Geometry check sheet. Reference: the model listing, model coordinates, mm. Face numbers are marked on the shaded views. A direction names the side the tool comes from. Round coordinates to 2 decimals unless told otherwise and drop trailing zeros. Order: outer loops, then holes, each group sorted by start corner. A loop starts at its lowest first (then second) coordinate and runs counter-clockwise, first axis right, second up.
(1) Set-up check for the marked faces 1 and 2: record each of +Z, -Z, +X, -X, +Y, -Y from which the full face is reachable in a straight line by a thin tool's end or side.
(2) Cross-section at C-C on x = -1. Enter the section's corners in (y, z) (3 decimals).
(3) Thickness scan on L1, parallel to Y at x = -2, z = -22.5 (3 decimals); L2, parallel to X at y = 26, z = -34; L3, parallel to Y at x = 6.25, z = -3.5 (3 decimals). Record the ranges inside material, lowest first.
(4) Gauge pin test, flat ends, axial feed: P1, Ø3.5, axis at y = 2.5, z = -10, coming from the -X side; P2, Ø5, axis at x = 7.5, z = -17, coming from the +Y side (3 decimals); P3, Ø10, axis at y = 6, z = -12.5, coming from the +X side. Record the tip position at first contact, or that the pin passes through.
(5) Cross-section at A-A on z = -11. Enter the section's corners in (x, y) (3 decimals), and give its area (3 significant figures).
(6) Draft check along X on the marked faces 3, 4 and 5. Enter one of: pulls with the +X half, pulls with the -X half, needs draft (parallel to the pull), parting line crosses it, or undercut.
from build123d import *
from build123d.topology import SkipClean

# Parameters (mm, degrees)
SKETCH1_W               = 12.7
SKETCH1_H               = 25.4
BOSS_EXTRUDE1_DEPTH     = 3.175
SKETCH17_W              = 12.7
SKETCH17_H              = 3.175
BOSS_EXTRUDE5_DEPTH     = 31.75
F_3_8_CLEARANCE_HOLE1_D = 10.31748
BOSS_EXTRUDE6_DEPTH     = 3.175
CUT_EXTRUDE4_DEPTH      = 52.789749346
SKETCH31_W              = 2.00025
SKETCH31_H              = 25.4
BOSS_EXTRUDE9_DEPTH     = 18.034
CUT_EXTRUDE6_DEPTH      = 54.550805677
CUT_EXTRUDE6_DEPTH_BACK = 54.550805677
BOSS_EXTRUDE10_START    = -3.175
BOSS_EXTRUDE10_DEPTH    = 3.175
BOSS_EXTRUDE11_START    = 3.175
BOSS_EXTRUDE11_DEPTH    = 3.175


with BuildPart() as part:
    # Sketch1 → Boss-Extrude1 (new body)
    with BuildSketch(Plane(origin=(0, 0, 0), x_dir=(1, 0, 0), z_dir=(0, 1, 0))):
        with Locations((0, 12.7)):
            Rectangle(SKETCH1_W, SKETCH1_H)
    extrude(amount=BOSS_EXTRUDE1_DEPTH)

    # Sketch17 → Boss-Extrude5 (add)
    with BuildSketch(Plane(origin=(0, 10.998522628, -6.35), x_dir=(-1, 0, 0), z_dir=(0, 0.866025403784438, -0.500000000000001))):
        with Locations((0, -20.409545256)):
            Rectangle(SKETCH17_W, SKETCH17_H)
    extrude(amount=BOSS_EXTRUDE5_DEPTH)

    # 3/8 Clearance Hole1 (through all)
    with Locations(Plane(origin=(0, -9.411022628, -16.300369343), x_dir=(1, 0, 0), z_dir=(0, 0.5000000000000011, 0.8660254037844379))):
        with Locations((0, 34.925)):
            Hole(F_3_8_CLEARANCE_HOLE1_D / 2)

    # Sketch26 → Boss-Extrude6 (add)
    with BuildSketch(Plane(origin=(0, -9.411022628, -16.300369343), x_dir=(1, 0, 0), z_dir=(0, 0.5000000000000011, 0.8660254037844379))):
        with BuildLine():
            ThreePointArc((6.35, 25.326635744), (10.137346679, 29.47657833), (11.50874, 34.925))
            ThreePointArc((11.50874, 34.925), (-5.44842167, 45.062346679), (-6.35, 25.326635744))
            Line((-6.35, 25.326635744), (-6.35, 44.45))
            Line((-6.35, 44.45), (6.35, 44.45))
            Line((6.35, 44.45), (6.35, 25.326635744))
        make_face()
    extrude(amount=-BOSS_EXTRUDE6_DEPTH)

    # Sketch27 → Cut-Extrude4 (cut, through all)
    with BuildSketch(Plane(origin=(0, 3.175, 0), x_dir=(1, 0, 0), z_dir=(0, 1, 0))):
        with BuildLine():
            Line((1.89865, 14.2875), (1.89865, 4.7625))
            ThreePointArc((1.89865, 4.7625), (0, 2.86385), (-1.89865, 4.7625))
            Line((-1.89865, 4.7625), (-1.89865, 14.2875))
            ThreePointArc((-1.89865, 14.2875), (0, 16.18615), (1.89865, 14.2875))
        make_face()
    extrude(amount=-CUT_EXTRUDE4_DEPTH, mode=Mode.SUBTRACT)

    # Sketch31 → Boss-Extrude9 (add)
    with BuildSketch(Plane.XZ):
        with Locations((-5.349875, -12.7)):
            Rectangle(SKETCH31_W, SKETCH31_H)
        with Locations((5.349875, -12.7)):
            Rectangle(SKETCH31_W, SKETCH31_H)
    extrude(amount=BOSS_EXTRUDE9_DEPTH)

    # Sketch32 → Cut-Extrude6 (cut, two sides: drawn at the far end of the back side and taken through both)
    with BuildSketch(Plane(origin=(0, 0, 0), x_dir=(0, 0, -1), z_dir=(1, 0, 0)).offset(-CUT_EXTRUDE6_DEPTH_BACK)):
        Polygon((0, -3.175), (23.566912895, -3.175), (25.4, 0), (41.090286181, -22.96252164), (-8.953256295, -22.624237032), align=None)
    extrude(amount=CUT_EXTRUDE6_DEPTH + CUT_EXTRUDE6_DEPTH_BACK, mode=Mode.SUBTRACT)

    # Sketch35 → Boss-Extrude10 (add)
    with BuildSketch(Plane(origin=(0, -10.998522628, -19.05), x_dir=(-1, 0, 0), z_dir=(0, -0.5000000000000012, -0.866025403784438)).offset(BOSS_EXTRUDE10_START)):
        with BuildLine():
            Line((-6.35, 9.033825791), (-11.26569769, 32.572309637))
            ThreePointArc((-11.26569769, 32.572309637), (-9.523820075, 28.463734832), (-6.35, 25.326635744))
            Line((-6.35, 25.326635744), (-6.35, 9.033825791))
        make_face()
        with BuildLine():
            Line((6.35, 9.033825791), (11.26569769, 32.572309637))
            ThreePointArc((11.26569769, 32.572309637), (9.523820075, 28.463734832), (6.35, 25.326635744))
            Line((6.35, 25.326635744), (6.35, 9.033825791))
        make_face()
    extrude(amount=BOSS_EXTRUDE10_DEPTH)

    # Sketch36 → Boss-Extrude11 (add)
    with SkipClean():  # the faces are left unmerged after this step: merging them gives an invalid solid
        with BuildSketch(Plane(origin=(0, -9.411022628, -16.300369343), x_dir=(1, 0, 0), z_dir=(0, 0.500000000000001, 0.8660254037844382)).offset(BOSS_EXTRUDE11_START)):
            with BuildLine():
                Line((-5.010829857, 15.04630998), (-4.471472861, 9.426131072))
                Line((-4.471472861, 9.426131072), (-6.35, 9.033825791))
                Line((-6.35, 9.033825791), (-11.26569769, 32.572309637))
                ThreePointArc((-11.26569769, 32.572309637), (0, 46.43374), (11.26569769, 32.572309637))
                Line((11.26569769, 32.572309637), (6.35, 9.033825791))
                Line((6.35, 9.033825791), (4.471472861, 9.426131072))
                Line((4.471472861, 9.426131072), (5.010829857, 15.04630998))
                Line((5.010829857, 15.04630998), (7.30501638, 26.031866015))
                ThreePointArc((7.30501638, 26.031866015), (0, 23.41626), (-7.30501638, 26.031866015))
                Line((-7.30501638, 26.031866015), (-5.010829857, 15.04630998))
            make_face()
            with BuildLine():
                ThreePointArc((-8.779337573, 33.09155271), (0, 25.95626), (8.779337573, 33.09155271))
                ThreePointArc((8.779337573, 33.09155271), (0, 43.89374), (-8.779337573, 33.09155271))
            make_face(mode=Mode.SUBTRACT)
        extrude(amount=-BOSS_EXTRUDE11_DEPTH)


solid = part.part
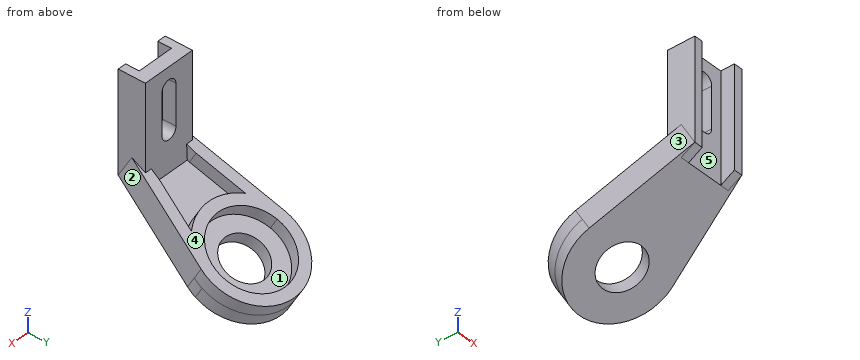
Found:
1. face 1: none
1. face 2: +Z, +X, -Y
2. outline: (0, -25.4) - (14.865, -33.982) - (16.452, -31.232) - (13.116, -29.306) - (14.704, -26.557) - (12.493, -25.281) - (10.906, -28.03) - (3.175, -23.567) - (3.175, -15.901) - (0, -15.901) - close; (0, -3.149) - (3.175, -3.149) - (3.175, 0) - (0, 0) - close; (23.63, -39.043) - (29.177, -42.245) - (32.352, -36.746) - (30.141, -35.47) - (28.554, -38.219) - (25.218, -36.293) - close
3. L1: y = 0 to 3.175
3. L2: x = -10.55 to -7.7, 7.7 to 10.55
3. L3: y = -3.175 to 3.175
4. P1: stops at x = -6.35
4. P2: stops at y = 3.175
4. P3: stops at x = 6.35
5. outline: (-6.35, -3.175) - (-4.35, -3.175) - (-4.35, 0) - (-1.899, 0) - (-1.899, 3.175) - (-6.35, 3.175) - close; (1.899, 0) - (4.35, 0) - (4.35, -3.175) - (6.35, -3.175) - (6.35, 3.175) - (1.899, 3.175) - close
5. area: 41.0 mm2
6. face 3: pulls with the -X half
6. face 4: needs draft
6. face 5: undercut
